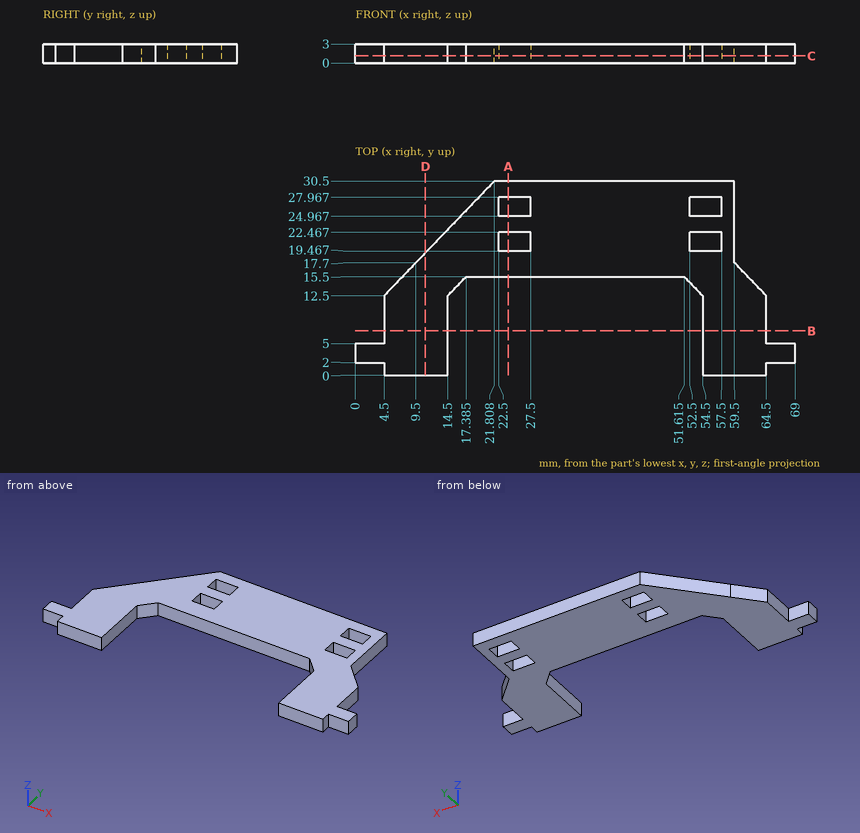
Can you work these out from the drawing? Everything is in mm from the part's minimum corner. Give positions to 0.01 mm unless a question says otherwise; leave off trailing zeros. Order: outer loops, then holes, each group sorted by start corner. A loop starts at its lowest first (then second) coordinate and runs counter-clockwise, first axis right, second up. Notation, with made-up numbers: M -21,36.25 L 29,36.25 A33 ccw 29,70.25 Z; hole C 70,72 d11. An arc over 180 degrees is marked long. One line per item, written item: value.
Item 1: If we section it at A-A on x = 24: Write out the boundary of the cut face in (y, z).
Verdict:
outline: M 15.5,0 L 19.47,0 L 19.47,3 L 15.5,3 Z; M 22.47,0 L 24.97,0 L 24.97,3 L 22.47,3 Z; M 27.97,0 L 30.5,0 L 30.5,3 L 27.97,3 Z
Item 2: For pin 1 (1.5 mm diameter, centred on y = 21, z = 1.5, fed in from +X); pin 2 (0.9 mm diameter, centred on x = 40.5, z = 1, fed in from -Y); pin 3 (1.5 mm diameter, centred on x = 2.5, z = 1, fed in from +Y), each with a flat end and sliding along its axis, tell me the tip position at first contact or that it passes through.
Verdict:
pin 1: x = 59.5
pin 2: y = 15.5
pin 3: y = 5
Item 3: Please list where these lines run through material, in increasing order: line 1 (Y direction, x = 57, z = 1.4); line 2 (X direction, y = 9, z = 0.5); line 3 (Y direction, x = 26, z = 1.2).
Verdict:
line 1: 0 to 19.47, 22.47 to 24.97, 27.97 to 30.5
line 2: 4.5 to 14.5, 54.5 to 64.5
line 3: 15.5 to 19.47, 22.47 to 24.97, 27.97 to 30.5
Item 4: If we section it at D-D on x = 11: Write out the boundary of the cut face in (y, z).
Verdict:
outline: M 0,0 L 19.26,0 L 19.26,3 L 0,3 Z
Item 5: If we section it at B-B on y = 7: Write out the boundary of the cut face in (x, z), and give its area (3 significant figures).
Verdict:
outline: M 4.5,0 L 14.5,0 L 14.5,3 L 4.5,3 Z; M 54.5,0 L 64.5,0 L 64.5,3 L 54.5,3 Z
area: 60.0 mm2
Item 6: If we section it at C-C on z = 1.15: State how many separate pieces and enclosed holes the cut face has, and give its area (3 significant figures).
Verdict:
separate pieces: 1
enclosed holes: 4
area: 953 mm2
